Drawing for the job (mm, zero at the part's lowest x, y, z). Give positions to 0.01 mm unless a question says otherwise; leave off trailing zeros. Write each loop counter-clockwise with the first axis right and the second up, starting at its lowest first coordinate (ties: lowest second). Pieces come first, ordered by that corner, then holes. Notation, with made-up numbers: M 79.5,86 L 92.5,86 A23 ccw 92.5,98 Z; hole C 45,45.5 d10. An arc over 180 degrees is marked long. Use a Markdown table: item, result. Add a question column.
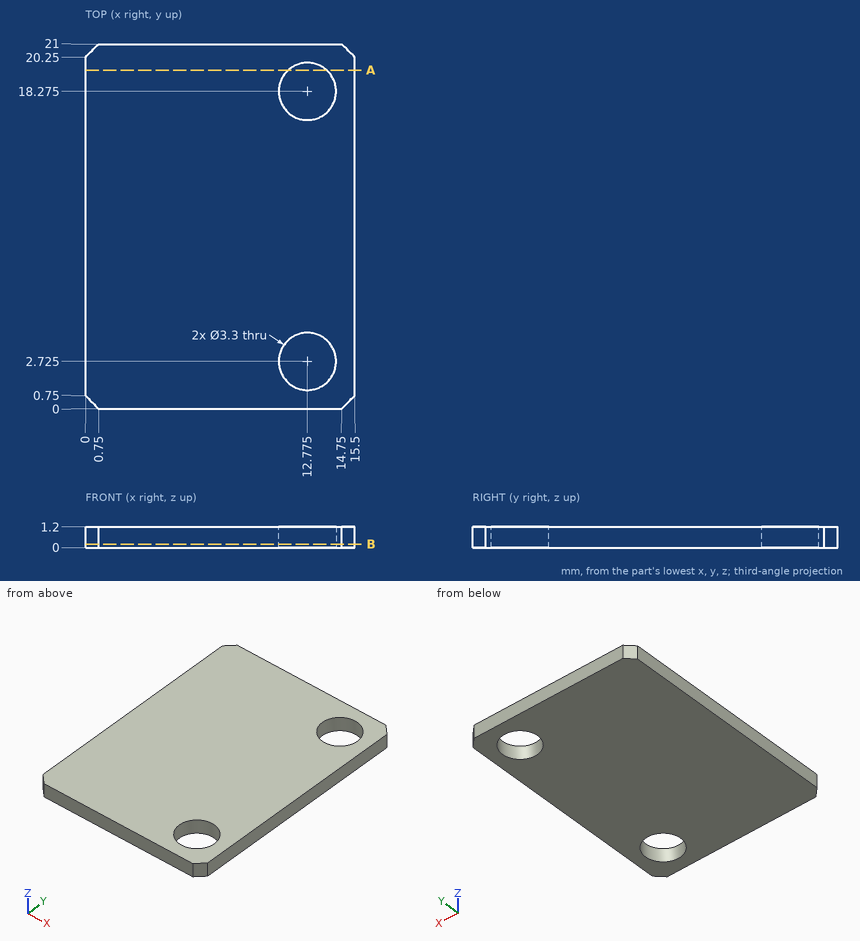
1. Cut at B-B (z = 0.2). Write the cut outline in (x, y) (3 decimals), then the cut area to 3 significant figures.
2. Drill centre lines: probe 1 along Y at (x, z) = (11.75, 0.95); probe 2 along Y at (x, z) = (14, 0.45); probe 3 along X at (y, z) = (17.75, 0.25). Where is each one in solid material? Low to high. Write a range as [from, to].
3. Cut at A-A (y = 19.5). Write the cut outline in (x, z).
4. Flat gauge pin, fed straight in: pin 1 (1.5 mm diameter, centred on x = 10, y = 12, fed in from -Z). Where does the tip first touch, or does it go through?
A:
| question | item | result |
|---|---|---|
| 1 | outline | M 0,0.75 L 0.75,0 L 14.75,0 L 15.5,0.75 L 15.5,20.25 L 14.75,21 L 0.75,21 L 0,20.25 Z; hole C 12.775,2.725 d3.3; hole C 12.775,18.275 d3.3 |
| 1 | area | 307 mm² |
| 2 | probe 1 | y = [0, 1.43], [4.02, 16.98], [19.57, 21] |
| 2 | probe 2 | y = [0, 1.62], [3.83, 17.17], [19.38, 21] |
| 2 | probe 3 | x = [0, 11.21], [14.34, 15.5] |
| 3 | outline | M 0,0 L 11.67,0 L 11.67,1.2 L 0,1.2 Z; M 13.88,0 L 15.5,0 L 15.5,1.2 L 13.88,1.2 Z |
| 4 | pin 1 | stops at z = 0 |
